Answer from the drawing. Dimensions are ordinates in mm from the lowest x, y and z of the part. Coordinates: 2 decimals unless noted, no trailing zeros. Loops run counter-clockwise (first coordinate to the right, second up) from the corner with the lowest first, then second, coordinate; pieces in that order, holes last.
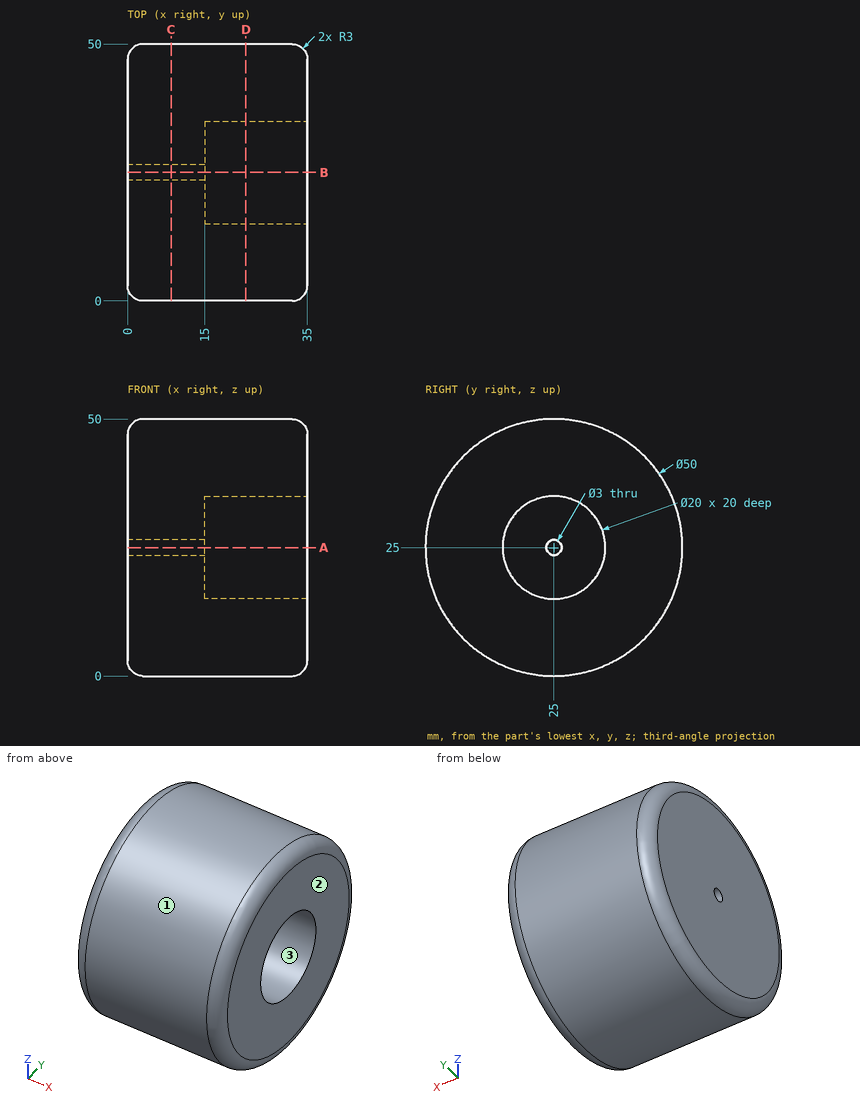
Item 1: A cutting plane is placed at D-D on x = 23. Determine the outline of the cut face in (y, z), then the cut area to 3 significant figures.
Numbers:
outline: circle Ø50 at (25, 25); hole circle Ø20 at (25, 25)
area: 1,650 mm2
Item 2: Find the intervals of material crossed by line 1 along Y through (x, z) = (29, 25); line 2 along Y through (x, z) = (5, 25); line 3 along X through (y, z) = (22.5, 33), in increasing order.
Numbers:
line 1: y = 0 to 15, 35 to 50
line 2: y = 0 to 23.5, 26.5 to 50
line 3: x = 0 to 15
Item 3: Given pin 1 (10 mm diameter, centred on x = 17.5, z = 14.5, fed in from +Y); pin 2 (3 mm diameter, centred on x = 23.5, y = 43.5, fed in from +Z); pin 3 (1 mm diameter, centred on x = 14.5, y = 26, fed in from -Z) (3 decimals), each flat-ended and moving along its own axis, determine where each tip first touches the part or whether it passes through.
Numbers:
pin 1: stops at y = 49.39
pin 2: stops at z = 43.33
pin 3: stops at z = 0.005
Item 4: A cutting plane is placed at A-A on z = 25. Determine the outline of the cut face in (x, y), then the cut area to 3 significant figures.
Numbers:
outline: (0, 3) arc R3 ccw to (3, 0) - (32, 0) arc R3 ccw to (35, 3) - (35, 15) - (15, 15) - (15, 23.5) - (0, 23.5) - close; (0, 26.5) - (15, 26.5) - (15, 35) - (35, 35) - (35, 47) arc R3 ccw to (32, 50) - (3, 50) arc R3 ccw to (0, 47) - close
area: 1,300 mm2
Item 5: Determine the mould class of the marked faces 1, 2 and 3 for opening direction Y: released by +Y, released by -Y, zero draft, split by the parting line, or undercut.
Numbers:
face 1: split by the parting line
face 2: zero draft
face 3: undercut
Item 6: A cutting plane is placed at C-C on x = 8.5. Determine the outline of the cut face in (y, z).
Numbers:
outline: circle Ø50 at (25, 25); hole circle Ø3 at (25, 25)
